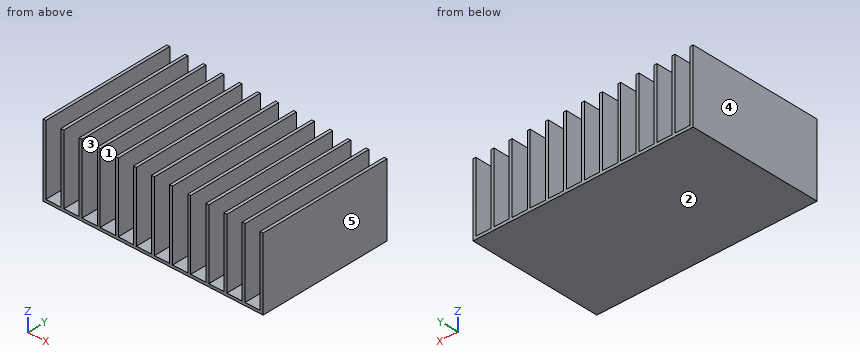
from build123d import *

# Parameters (mm, degrees)
F0_W     = 1930.4
F0_H     = 1168.4
F1_DEPTH = 25.4
F2_W     = 25.4
F2_H     = 1168.4
F3_DEPTH = 609.6


with BuildPart() as f1:
    # F0 (on Top) → F1 (new body)
    with BuildSketch(Plane.XY):
        Rectangle(F0_W, F0_H)
    extrude(amount=F1_DEPTH)

    # F2 (on face) → F3 (join)
    with BuildSketch(Plane.XY.offset(25.4)):
        with Locations((-952.5, 0)):
            Rectangle(F2_W, F2_H)
        with Locations((-793.75, 0)):
            Rectangle(F2_W, F2_H)
        with Locations((-635, 0)):
            Rectangle(F2_W, F2_H)
        with Locations((-476.25, 0)):
            Rectangle(F2_W, F2_H)
        with Locations((-317.5, 0)):
            Rectangle(F2_W, F2_H)
        with Locations((-158.75, 0)):
            Rectangle(F2_W, F2_H)
        Rectangle(F2_W, F2_H)
        with Locations((158.75, 0)):
            Rectangle(F2_W, F2_H)
        with Locations((317.5, 0)):
            Rectangle(F2_W, F2_H)
        with Locations((476.25, 0)):
            Rectangle(F2_W, F2_H)
        with Locations((635, 0)):
            Rectangle(F2_W, F2_H)
        with Locations((793.75, 0)):
            Rectangle(F2_W, F2_H)
        with Locations((952.5, 0)):
            Rectangle(F2_W, F2_H)
    extrude(amount=F3_DEPTH)


solid = f1.part
Check sheet for the modelled part. Datum: model origin and axes. Units: mm. Face numbers are marked on the shaded views. A direction names the side the tool comes from. Coordinates: 2 decimals unless noted, no trailing zeros. Write each loop counter-clockwise with the first axis right and the second up, starting at its lowest first coordinate (ties: lowest second). Pieces come first, ordered by that corner, then holes. Notation, with made-up numbers: M -15,4.25 L -11,4.25 A27 cw -11,29.25 Z; hole C -30.75,48 d6. An arc over 180 degrees is marked long. Answer as CSV lines item,"result".
Q1. Mould release check, pull along X, two halves, no side actions. Record for the marked faces 3, 4 and 5: released by +X, released by -X, zero draft, split by the parting line, or undercut.
Check result:
face 3,"undercut"
face 4,"released by -X"
face 5,"released by +X"
Q2. Set-up check for the marked faces 1 and 2: record each of +Z, -Z, +X, -X, +Y, -Y from which the full face is reachable in a straight line by a thin tool's end or side.
Check result:
face 1,"+Z, +Y, -Y"
face 2,"-Z, +X, -X, +Y, -Y"
Q3. Material ranges on probe 1 along Z at (x, y) = (125, -87), recorded low to high. Write a range as from..to.
Check result:
probe 1,"0..25.4"
Q4. Cross-section at B-B (x = -46.5). Record the boundary of the cut face in (y, z), then the cut area to 3 significant figures.
Check result:
outline,"M -584.2,0 L 584.2,0 L 584.2,25.4 L -584.2,25.4 Z"
area,"29,700 mm^2"
Q5. Cross-section at A-A (z = 233.5). Count the separate pieces of the cut face and the enclosed holes in it, then the cut area to 3 significant figures.
Check result:
separate pieces,"13"
enclosed holes,"0"
area,"386,000 mm^2"
